Geometry: see drawing. Coordinates: mm, zero at the bounding-box minimum. A direction names the side the tool comes from. Coordinates: 2 decimals unless noted, no trailing zeros. Write each loop counter-clockwise with the first axis right and the second up, starting at its lowest first coordinate (ties: lowest second). Pieces come first, ordered by that corner, then holes. Notation, with made-up numbers: M 4,32.5 L 62,32.5 A21 ccw 62,58.5 Z; hole C -9,57 d10. An arc over 180 degrees is marked long. One line per item, written item: value. Start each with the question number.
Item 1: Mould query, pull axis Z, two halves, no side actions, for the marked faces 3, 4 and 5. Classes: released by +Z, released by -Z, zero draft, split by the parting line, or undercut.
Item 2: Set-up query: the marked faces 1 and 2. Return all of +Z, -Z, +X, -X, +Y, -Y with unobstructed straight access to the full face (end or side cutting, diameter ignored); none if empty.
Item 3: Cut plane B-B, the plane z = 10.9. Output: boundary loops of the cut face in (x, y) (3 decimals).
Item 4: Pin query (flat end, axial travel): P1, Ø1.5, axis at x = 11.5, y = 8, coming from the -Z side (3 decimals); P2, Ø4, axis at y = 4.5, z = 15, coming from the +X side; P3, Ø2, axis at x = 7, y = 3, coming from the +Z side. Return the tip coordinate at first contact, or that it passes through.
Item 5: Cut plane A-A, the plane x = 10.9. Output: boundary loops of the cut face in (y, z) (3 decimals).
Item 6: Ray query, L1, parallel to X at y = 10.75, z = 10.9 (3 decimals); L2, parallel to X at y = 19.25, z = 10.25; L3, parallel to Z at x = 6.25, y = 1.75. Return the intervals inside material, ascending. Write a range as from..to.
Item 7: Cut plane C-C, the plane y = 19.25. State how many separate pieces and enclosed holes the cut face has, then the cut area to 3 significant figures.
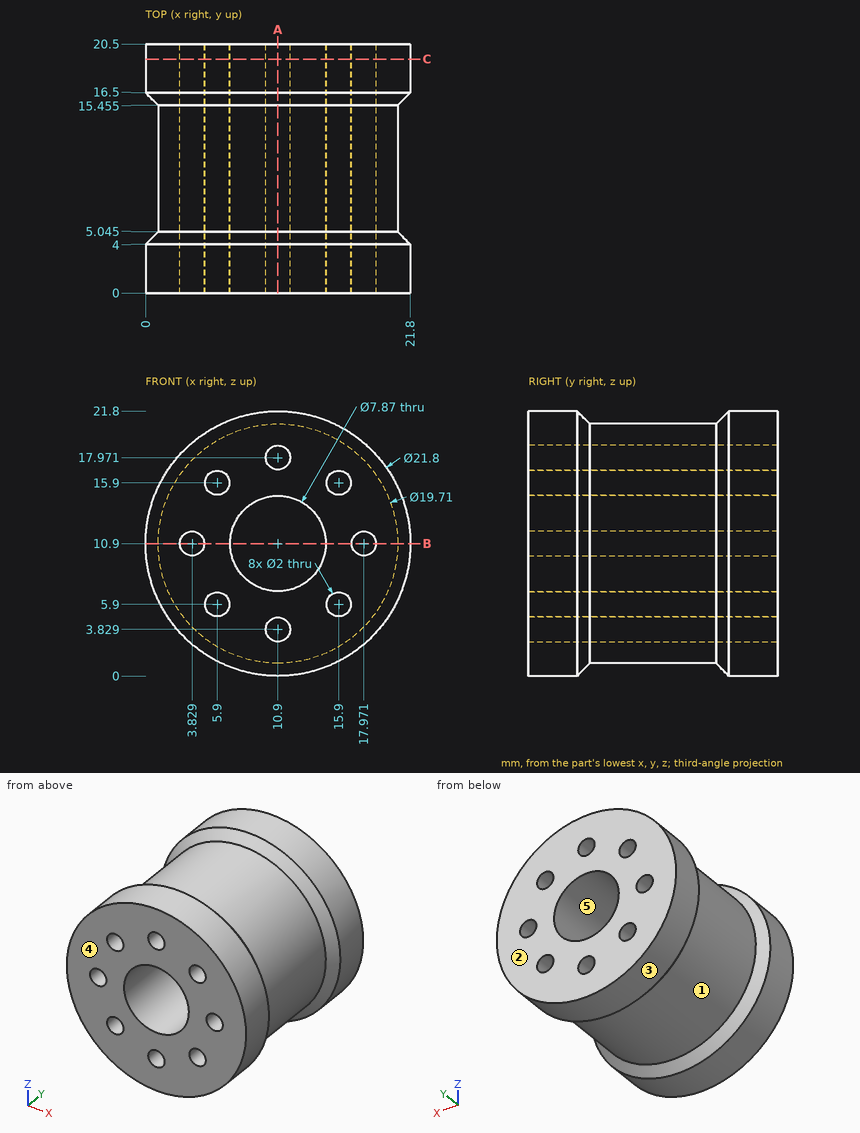
From the geometry:
1. face 3: split by the parting line
1. face 4: zero draft
1. face 5: undercut
2. face 1: none
2. face 2: +Z, -Z, +X, -X, +Y
3. outline: M 0,0 L 2.829,0 L 2.829,20.5 L 0,20.5 L 0,16.5 L 1.045,15.455 L 1.045,5.045 L 0,4 Z; M 4.829,0 L 6.965,0 L 6.965,20.5 L 4.829,20.5 Z; M 14.835,0 L 16.971,0 L 16.971,20.5 L 14.835,20.5 Z; M 18.971,0 L 21.8,0 L 21.8,4 L 20.755,5.045 L 20.755,15.455 L 21.8,16.5 L 21.8,20.5 L 18.971,20.5 Z
4. P1: stops at z = 1.045
4. P2: stops at x = 21.58
4. P3: stops at z = 21.41
5. outline: M 0,0 L 4,0 L 5.045,1.045 L 15.455,1.045 L 16.5,0 L 20.5,0 L 20.5,2.829 L 0,2.829 Z; M 0,4.829 L 20.5,4.829 L 20.5,6.965 L 0,6.965 Z; M 0,14.835 L 20.5,14.835 L 20.5,16.971 L 0,16.971 Z; M 0,18.971 L 20.5,18.971 L 20.5,21.8 L 16.5,21.8 L 15.455,20.755 L 5.045,20.755 L 4,21.8 L 0,21.8 Z
6. L1: x = 1.045..2.829, 4.829..6.965, 14.835..16.971, 18.971..20.755
6. L2: x = 0.02..3.07, 4.59..7.02, 14.78..17.21, 18.73..21.78
6. L3: z = 1.04..4.96, 6.84..14.96, 16.84..20.76
7. separate pieces: 1
7. enclosed holes: 9
7. area: 299 mm²
